Can you work these out from the drawing? Everything is in mm from the part's minimum corner. A direction names the side the tool comes from. Coordinates: 2 decimals unless noted, no trailing zeros. Order: outer loops, then holes, each group sorted by start corner. A loop starts at its lowest first (then second) coordinate and runs counter-clockwise, first axis right, second up. Notation, with made-up numbers: (43, 88.25) -> (56, 88.25) arc R32 cw to (56, 115.25) -> close; hole circle Ø1 at (13.5, 35.25). An arc over 180 degrees is marked (long way). Use a Markdown table: item, result. Add a question column.
1) If we section it at C-C (z = 8.75): Write out the boundary of the cut face in (x, y), plus the area to 3 significant figures.
2) Which directions (+Z, -Z, +X, -X, +Y, -Y) give clear straight access to the entire face, cutting with the end or side of a thin tool? Please do the marked faces 1, 2, 3 and 4.
3) If we section it at B-B (x = 11.3): Write out the boundary of the cut face in (y, z), plus the area to 3 significant figures.
4) If we section it at D-D (y = 32.5): Write out the boundary of the cut face in (x, z).
5) If we section it at A-A (x = 28.5): Write out the boundary of the cut face in (y, z), plus the area to 3 significant figures.
6) If I drill on L1, parallel to Y at x = 12, z = 14.5; L2, parallel to Y at x = 23.5, z = 9; L3, parallel to Y at x = 12.5, z = 9.5, over which ranges is the centre line in solid material (lowest first)? Write a range as [from, to].
7) Will these pins go through, and if not, where does the flat tip stop? pin 1 Ø6 at (x, y) = (14.5, 20) entering from -Z; pin 2 Ø2 at (x, z) = (31, 3.5) entering from -Y; pin 3 Ø6 at (x, z) = (26.5, 12.5) entering from +Y; pin 4 Ø8 at (x, z) = (24.5, 4.5) entering from -Y.
8) Thinking about a two-plate mould opening in Y: for the marked faces 5, 6, 7 and 8, which applies, +Y half, -Y half, draft (parallel to the pull), parting line (faces both ways), or undercut?
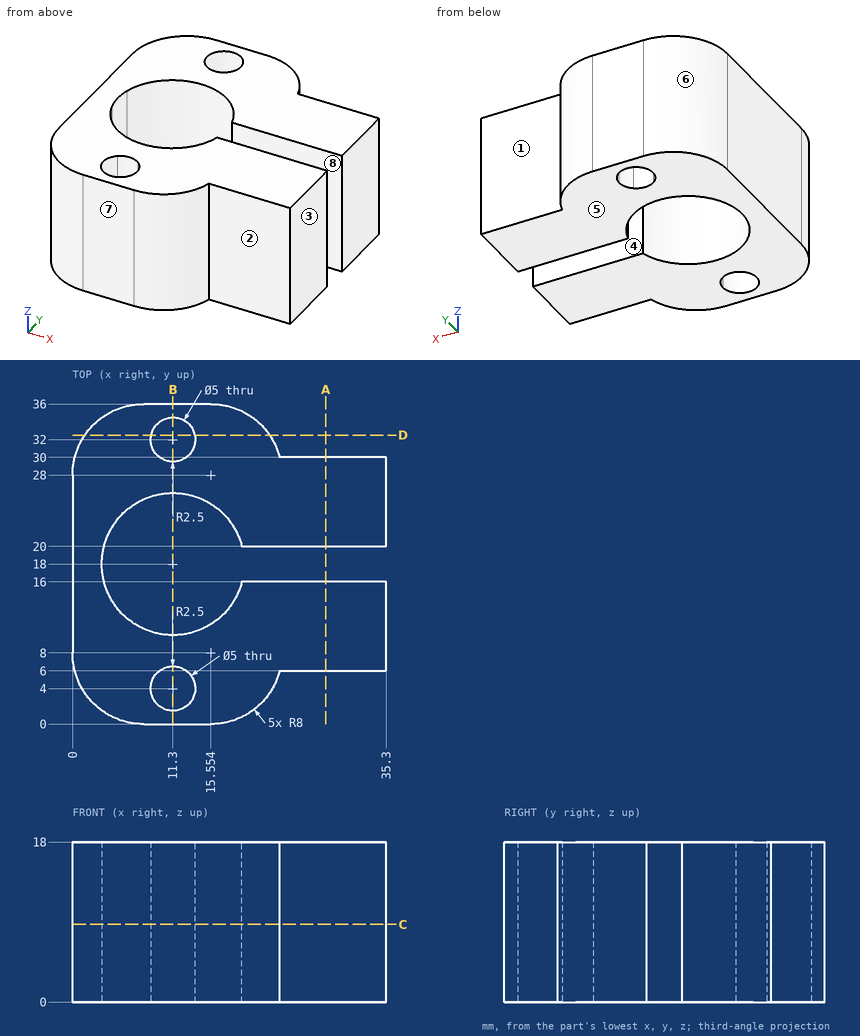
Answer sheet:
| question | item | result |
|---|---|---|
| 1 | outline | (0, 8) arc R8 ccw to (8, 0) -> (15.55, 0) arc R8 ccw to (23.3, 6) -> (35.3, 6) -> (35.3, 16) -> (19.05, 16) arc R8 cw (long way) to (19.05, 20) -> (35.3, 20) -> (35.3, 30) -> (23.3, 30) arc R8 ccw to (15.55, 36) -> (8, 36) arc R8 ccw to (0, 28) -> close; hole circle Ø5 at (11.3, 4); hole circle Ø5 at (11.3, 32) |
| 1 | area | 771 mm2 |
| 2 | face 1 | +Z, -Z, +X, +Y |
| 2 | face 2 | +Z, -Z, +X, -Y |
| 2 | face 3 | +Z, -Z, +X, +Y, -Y |
| 2 | face 4 | +Z, -Z, +X |
| 3 | outline | (0, 0) -> (1.5, 0) -> (1.5, 18) -> (0, 18) -> close; (6.5, 0) -> (10, 0) -> (10, 18) -> (6.5, 18) -> close; (26, 0) -> (29.5, 0) -> (29.5, 18) -> (26, 18) -> close; (34.5, 0) -> (36, 0) -> (36, 18) -> (34.5, 18) -> close |
| 3 | area | 180 mm2 |
| 4 | outline | (1.39, 0) -> (8.85, 0) -> (8.85, 18) -> (1.39, 18) -> close; (13.75, 0) -> (22.17, 0) -> (22.17, 18) -> (13.75, 18) -> close |
| 5 | outline | (6, 0) -> (16, 0) -> (16, 18) -> (6, 18) -> close; (20, 0) -> (30, 0) -> (30, 18) -> (20, 18) -> close |
| 5 | area | 360 mm2 |
| 6 | L1 | [0, 1.6], [6.4, 10.03], [25.97, 29.6], [34.4, 36] |
| 6 | L2 | [6, 16], [20, 30] |
| 6 | L3 | [0, 1.81], [6.19, 10.09], [25.91, 29.81], [34.19, 36] |
| 7 | pin 1 | through |
| 7 | pin 2 | y = 6 |
| 7 | pin 3 | y = 30 |
| 7 | pin 4 | y = 1.71 |
| 8 | face 5 | draft |
| 8 | face 6 | +Y half |
| 8 | face 7 | -Y half |
| 8 | face 8 | undercut |
